Read the model definition and answer for the solid it produces. Units are mm, in the model's axes. A direction names the side the tool comes from. Coordinates: 2 decimals unless noted, no trailing zeros. Write each loop counter-clockwise with the first axis right and the second up, starting at its lowest first coordinate (ties: lowest second). Pieces come first, ordered by that corner, then holes.
1) Which of the six approach directions +Z, -Z, +X, -X, +Y, -Y give full straight-line access (tool end or side, diameter ignored) to faces 1 (the face through (-5, 10, 0)), 2 (the face through (-7, -47, 1)), 3 (the face through (-7, 65, 1)), 4 (the face through (0, 26, 1))?
2) The part is cut by section B-B (z = 1.1). Give the number of separate pieces and of enclosed holes in the cut face, then the cut area to 3 significant figures.
3) Each of these flat-tipped pins is pushed along its axis until it touches: pin 1 Ø0.9 at (x, z) = (-1.5, 2) entering from +Y; pin 2 Ø0.9 at (y, z) = (-48, 2) entering from +X; pin 3 Ø1.5 at (y, z) = (-44, 1) entering from +X. Where does it stop, or does it pass through?
4) Determine the mould class of faces 5 (the face through (2, 70, 1)), 6 (the face through (-3, 65, 1)), 7 (the face through (-15, -51, 1)) for opening direction X: +X half, -X half, draft (parallel to the pull), parting line (faces both ways), or undercut.
5) Find the intervals of material crossed by line 1 (Y direction, x = -2.5, z = 1.05); line 2 (X direction, y = 54.5, z = 1.9); line 3 (X direction, y = -9, z = 2.35), in increasing order.
6) The part is cut by section A-A (x = -4.5). Determine the outline of the cut face in (y, z), then the cut area to 4 significant figures.
from build123d import *

# Parameters (mm, degrees)
CROQUIS1_W              = 10
CROQUIS1_H              = 3
SALIENTE_EXTRUIR1_DEPTH = 3


with BuildPart() as part:
    # Croquis1 → Saliente-Extruir1 (new body)
    with BuildSketch(Plane.XY):
        with BuildLine():
            Line((-10, 70), (-10, 67))
            Line((-10, 67), (-7, 67))
            Line((-7, 67), (-7, 63))
            Line((-7, 63), (-9.5, 63))
            Line((-9.5, 63), (-9.5, 60))
            Line((-9.5, 60), (-0.5, 60))
            Line((-0.5, 60), (-0.5, 63))
            Line((-0.5, 63), (-3, 63))
            Line((-3, 63), (-3, 67))
            Line((-3, 67), (0, 67))
            Line((0, 67), (0, 70))
            Line((0, 70), (5, 70))
            Line((5, 70), (5, 67.405747627))
            ThreePointArc((5, 67.405747627), (4.929306729, 67.036438809), (4.727221995, 66.719345288))
            add(Edge.make_bspline(
                [(4.727221995, 66.719345288), (3.242407332, 65.146230192), (1.757592668, 62), (3.242407332, 58.853769808), (4.727221995, 57.280654712)],
                knots=[0.028065471, 0.028065471, 0.028065471, 0.028065471, 0.5, 0.971934529, 0.971934529, 0.971934529, 0.971934529], degree=3))
            ThreePointArc((4.727221995, 57.280654712), (4.929306729, 56.963561191), (5, 56.594252373))
            Line((5, 56.594252373), (5, 54.181314171))
            ThreePointArc((5, 54.181314171), (4.9841425, 54.003934523), (4.937072921, 53.832180471))
            add(Edge.make_bspline(
                [(4.937072921, 53.832180471), (3.31235764, 49.471453647), (1.68764236, 40.75), (3.31235764, 32.028546353), (4.937072921, 27.667819529)],
                knots=[0.006332812, 0.006332812, 0.006332812, 0.006332812, 0.5, 0.993667188, 0.993667188, 0.993667188, 0.993667188], degree=3))
            ThreePointArc((4.937072921, 27.667819529), (4.9841425, 27.496065477), (5, 27.318685829))
            Line((5, 27.318685829), (5, 24.567654138))
            ThreePointArc((5, 24.567654138), (4.997723384, 24.500214919), (4.990903903, 24.433082766))
            add(Edge.make_bspline(
                [(4.990903903, -48.933082766), (3.330301301, -36.70538851), (1.669698699, -12.25), (3.330301301, 12.20538851), (4.990903903, 24.433082766)],
                knots=[0.000910439, 0.000910439, 0.000910439, 0.000910439, 0.5, 0.999089561, 0.999089561, 0.999089561, 0.999089561], degree=3))
            ThreePointArc((4.990903903, -48.933082766), (4.997723384, -49.000214919), (5, -49.067654138))
            Line((5, -49.067654138), (5, -51.701381229))
            Line((5, -51.701381229), (5, -52))
            Line((5, -52), (0, -52))
            Line((0, -52), (0, -49))
            Line((0, -49), (-3, -49))
            Line((-3, -49), (-3, -45.5))
            Line((-3, -45.5), (-0.5, -45.5))
            Line((-0.5, -45.5), (-0.5, -42.5))
            Line((-0.5, -42.5), (-9.5, -42.5))
            Line((-9.5, -42.5), (-9.5, -45.5))
            Line((-9.5, -45.5), (-7, -45.5))
            Line((-7, -45.5), (-7, -49))
            Line((-7, -49), (-10, -49))
            Line((-10, -49), (-10, -52))
            Line((-10, -52), (-15, -52))
            Line((-15, -52), (-15, -51.701381229))
            Line((-15, -51.701381229), (-15, -49.067654138))
            ThreePointArc((-15, -49.067654138), (-14.997723384, -49.000214919), (-14.990903903, -48.933082766))
            add(Edge.make_bspline(
                [(-14.990903903, -48.933082766), (-13.330301301, -36.70538851), (-11.669698699, -12.25), (-13.330301301, 12.20538851), (-14.990903903, 24.433082766)],
                knots=[0.000910439, 0.000910439, 0.000910439, 0.000910439, 0.5, 0.999089561, 0.999089561, 0.999089561, 0.999089561], degree=3))
            ThreePointArc((-14.990903903, 24.433082766), (-14.997723384, 24.500214919), (-15, 24.567654138))
            Line((-15, 24.567654138), (-15, 27.318685829))
            ThreePointArc((-15, 27.318685829), (-14.9841425, 27.496065477), (-14.937072921, 27.667819529))
            add(Edge.make_bspline(
                [(-14.937072921, 53.832180471), (-13.31235764, 49.471453647), (-11.68764236, 40.75), (-13.31235764, 32.028546353), (-14.937072921, 27.667819529)],
                knots=[0.006332812, 0.006332812, 0.006332812, 0.006332812, 0.5, 0.993667188, 0.993667188, 0.993667188, 0.993667188], degree=3))
            ThreePointArc((-14.937072921, 53.832180471), (-14.9841425, 54.003934523), (-15, 54.181314171))
            Line((-15, 54.181314171), (-15, 56.594252373))
            ThreePointArc((-15, 56.594252373), (-14.929306729, 56.963561191), (-14.727221995, 57.280654712))
            add(Edge.make_bspline(
                [(-14.727221995, 57.280654712), (-13.242407332, 58.853769808), (-11.757592668, 62), (-13.242407332, 65.146230192), (-14.727221995, 66.719345288)],
                knots=[0.028065471, 0.028065471, 0.028065471, 0.028065471, 0.5, 0.971934529, 0.971934529, 0.971934529, 0.971934529], degree=3))
            ThreePointArc((-14.727221995, 66.719345288), (-14.929306729, 67.036438809), (-15, 67.405747627))
            Line((-15, 67.405747627), (-15, 70))
            Line((-15, 70), (-10, 70))
        make_face()
        with Locations((-5, 26)):
            Rectangle(CROQUIS1_W, CROQUIS1_H, mode=Mode.SUBTRACT)
        with Locations((-5, 55.5)):
            Rectangle(CROQUIS1_W, CROQUIS1_H, mode=Mode.SUBTRACT)
    extrude(amount=SALIENTE_EXTRUIR1_DEPTH)


solid = part.part
Reported:
1. face 1: -Z, +X, -X, +Y, -Y
1. face 2: +Z, -Z, -Y
1. face 3: +Z, -Z, +Y
1. face 4: +Z, -Z
2. separate pieces: 1
2. enclosed holes: 2
2. area: 1,870 mm2
3. pin 1: stops at y = 67
3. pin 2: stops at x = 4.93
3. pin 3: stops at x = 4.46
4. face 5: draft
4. face 6: undercut
4. face 7: -X half
5. line 1: y = -49 to -45.5, -42.5 to 24.5, 27.5 to 54, 57 to 60, 63 to 67
5. line 2: x = -15 to -10, 0 to 5
5. line 3: x = -12.52 to 2.52
6. outline: (-42.5, 0) - (24.5, 0) - (24.5, 3) - (-42.5, 3) - close; (27.5, 0) - (54, 0) - (54, 3) - (27.5, 3) - close; (57, 0) - (60, 0) - (60, 3) - (57, 3) - close
6. area: 289.5 mm2
